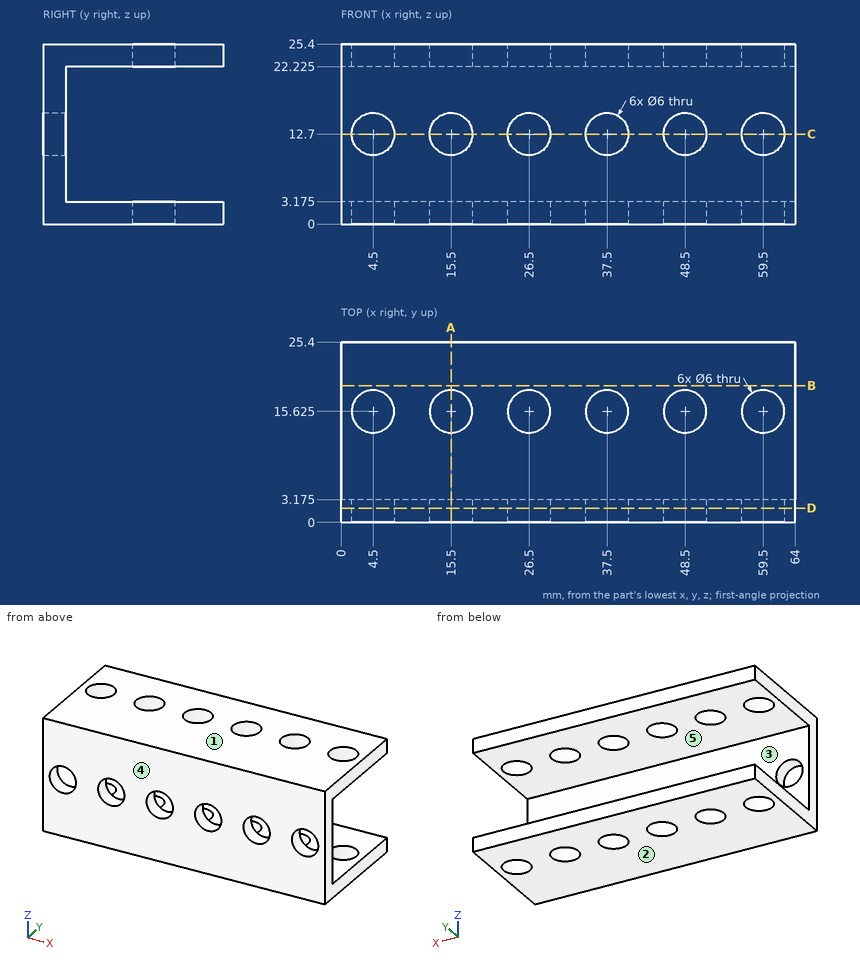
Here's the drawing with two shaded views (mm, measured from the low corner). I have some questions. A direction names the side the tool comes from. Coordinates: 2 decimals unless noted, no trailing zeros. Loops run counter-clockwise (first coordinate to the right, second up) from the corner with the lowest first, then second, coordinate; pieces in that order, holes last. Notation, with made-up numbers: (88.25, 32.5) - (128.25, 32.5) arc R32 cw to (128.25, 64.5) - close; hole circle Ø1 at (84, 83.5). An arc over 180 degrees is marked (long way). Answer as CSV lines item,"result". Start each with the question number.
1) Thinking about a two-plate mould opening in Z: for the marked faces 1, 2 and 3, which applies, pulls with the +Z half, pulls with the -Z half, needs draft (parallel to the pull), parting line crosses it, or undercut?
2) Suppose I cut it at C-C (z = 12.7). Please give me the cut outline in (x, y) (3 decimals).
3) Suppose I cut it at D-D (y = 2). Please give me the cut outline in (x, z).
4) Which directions (+Z, -Z, +X, -X, +Y, -Y) give clear straight access to the entire face, cutting with the end or side of a thin tool? Please do the marked faces 4 and 5.
5) Suppose I cut it at A-A (x = 15.5). Please give me the cut outline in (y, z) (3 decimals), plus the area to 3 significant figures.
6) Suppose I cut it at B-B (y = 19.25). Please give me the cut outline in (x, z) (3 decimals), plus the area to 3 significant figures.
7) I need wall thicknesses on line 1 (Z direction, x = 41.5, y = 9.25) (3 decimals); line 2 (Y direction, x = 59.5, z = 1.7) (3 decimals); line 3 (Z direction, x = 37.5, y = 2.4). Which ranges of each line are inside material? Lowest first, please. Write a range as from..to.
8) For pin 1 (9.5 mm diameter, centred on x = 23.5, z = 11.5, fed in from +Y) (3 decimals); pin 2 (5.5 mm diameter, centred on x = 4.5, z = 12.7, fed in from -Y), each with a flat end and sliding along its axis, tell me the tip position at first contact or that it passes through.
Check result:
1,face 1,"pulls with the +Z half"
1,face 2,"pulls with the -Z half"
1,face 3,"undercut"
2,outline,"(0, 0) - (1.5, 0) - (1.5, 3.175) - (0, 3.175) - close; (7.5, 0) - (12.5, 0) - (12.5, 3.175) - (7.5, 3.175) - close; (18.5, 0) - (23.5, 0) - (23.5, 3.175) - (18.5, 3.175) - close; (29.5, 0) - (34.5, 0) - (34.5, 3.175) - (29.5, 3.175) - close; (40.5, 0) - (45.5, 0) - (45.5, 3.175) - (40.5, 3.175) - close; (51.5, 0) - (56.5, 0) - (56.5, 3.175) - (51.5, 3.175) - close; (62.5, 0) - (64, 0) - (64, 3.175) - (62.5, 3.175) - close"
3,outline,"(0, 0) - (64, 0) - (64, 25.4) - (0, 25.4) - close; hole circle Ø6 at (4.5, 12.7); hole circle Ø6 at (15.5, 12.7); hole circle Ø6 at (26.5, 12.7); hole circle Ø6 at (37.5, 12.7); hole circle Ø6 at (48.5, 12.7); hole circle Ø6 at (59.5, 12.7)"
4,face 4,"+Z, -Z, +X, -X, -Y"
4,face 5,"+X, -X, +Y"
5,outline,"(0, 0) - (12.625, 0) - (12.625, 3.175) - (3.175, 3.175) - (3.175, 9.7) - (0, 9.7) - close; (0, 15.7) - (3.175, 15.7) - (3.175, 22.225) - (12.625, 22.225) - (12.625, 25.4) - (0, 25.4) - close; (18.625, 0) - (25.4, 0) - (25.4, 3.175) - (18.625, 3.175) - close; (18.625, 22.225) - (25.4, 22.225) - (25.4, 25.4) - (18.625, 25.4) - close"
5,area,"165 mm²"
6,outline,"(0, 0) - (64, 0) - (64, 3.175) - (0, 3.175) - close; (0, 22.225) - (64, 22.225) - (64, 25.4) - (0, 25.4) - close"
6,area,"406 mm²"
7,line 1,"z = 0..3.175, 22.225..25.4"
7,line 2,"y = 0..12.625, 18.625..25.4"
7,line 3,"z = 0..9.7, 15.7..25.4"
8,pin 1,"stops at y = 3.175"
8,pin 2,"passes through"
